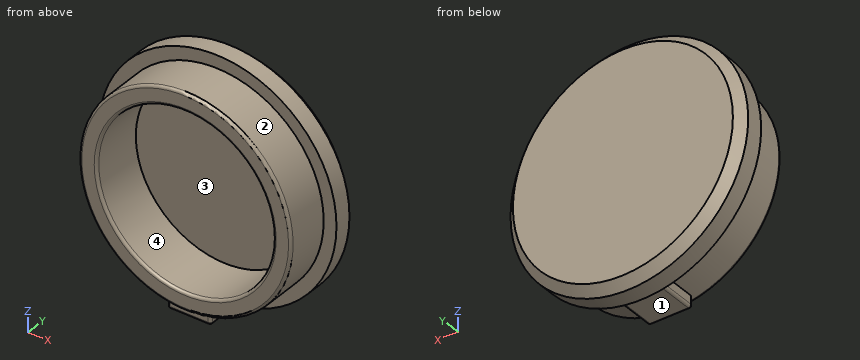
```python
from build123d import *

# Parameters (mm, degrees)
F0_R          = 12
F0_R_2        = 10
F1_DEPTH      = 6
F2_R          = 13.45
F3_DEPTH      = 1
F3_DEPTH_BACK = 2
F4_R          = 10
F5_DEPTH      = 6
F6_W          = 4.9
F6_H          = 2
F7_DEPTH      = 5.4
F8_SIZE       = 1
F9_R          = 0.3
F10_R         = 0.3


with BuildPart() as f1:
    # F0 (on Front) → F1 (new body)
    with BuildSketch(Plane.XZ):
        Circle(F0_R)
        Circle(F0_R_2, mode=Mode.SUBTRACT)
    extrude(amount=F1_DEPTH)

    # F2 (on Front) → F3 (join, two sides)
    with BuildSketch(Plane.XZ) as f3_sk:
        Circle(F2_R)
    extrude(amount=F3_DEPTH)
    extrude(f3_sk.sketch, amount=-F3_DEPTH_BACK)

    # F4 (on Front) → F5 (cut, through all)
    with BuildSketch(Plane.XZ):
        Circle(F4_R)
    extrude(amount=F5_DEPTH, mode=Mode.SUBTRACT)

    # F6 (on Front) → F7 (join)
    with BuildSketch(Plane.XZ):
        with Locations((0, -12)):
            Rectangle(F6_W, F6_H)
    extrude(amount=F7_DEPTH)

    # F8
    f8_edges = [f1.edges().sort_by_distance(p)[0] for p in [
        (-13.45, 2, 0),
    ]]
    chamfer(f8_edges, length=F8_SIZE)

    # F9
    f9_edges = [f1.edges().sort_by_distance(p)[0] for p in [
        (-2.45, -3.2, -13),
        (0, -5.4, -13),
        (2.45, -3.2, -13),
        (-2.45, -5.4, -12.373617),
        (2.45, -5.4, -12.373617),
    ]]
    fillet(f9_edges, radius=F9_R)

    # F10
    f10_edges = [f1.edges().sort_by_distance(p)[0] for p in [
        (-12, -6, 0),
        (-10, -6, 0),
    ]]
    fillet(f10_edges, radius=F10_R)


solid = f1.part
```
Geometry check sheet. Reference: the model listing, model coordinates, mm. Face numbers are marked on the shaded views. Round coordinates to 2 decimals unless told otherwise and drop trailing zeros. Order: outer loops, then holes, each group sorted by start corner. A loop starts at its lowest first (then second) coordinate and runs counter-clockwise, first axis right, second up. Notation, with made-up numbers: (-7, 68.5) - (23, 68.5) arc R19 cw to (23, 101.5) - close; hole circle Ø3 at (47.5, 34). An arc over 180 degrees is marked (long way). Use a Markdown table: item, result. Add a question column.
1) Mould release check, pull along X, two halves, no side actions. Record for the marked faces 1, 2, 3 and 4: released by +X, released by -X, zero draft, split by the parting line, or undercut.
2) Thickness scan on line 1 along Z through (x, y) = (0, -4.1); line 2 along Y through (x, z) = (11.5, -4.5); line 3 along X through (y, z) = (-1.25, -12.5). Record the ranges inside material, lowest first.
3) Section check B-B (y = -4.5). Record the cut outline in (x, z).
4) Section check C-C (z = 0). Record the cut outline in (x, y), then the cut area to 3 significant figures.
5) Gauge pin test, flat ends, axial feed: P1, Ø2, axis at y = -2.5, z = 8, coming from the -X side; P2, Ø3.5, axis at x = -0.5, y = -3.5, coming from the -Z side; P3, Ø0.8, axis at y = -2.5, z = -12.5, coming from the -X side. Record the tip position at first contact, or that the pin passes through.
6) Section check A-A (x = 0). Record the cut outline in (y, z), then the cut area to 3 significant figures.
Established:
| question | item | result |
|---|---|---|
| 1 | face 1 | zero draft |
| 1 | face 2 | split by the parting line |
| 1 | face 3 | undercut |
| 1 | face 4 | undercut |
| 2 | line 1 | -13 to -10, 10 to 12 |
| 2 | line 2 | -1 to 2 |
| 2 | line 3 | -2.45 to 2.45 |
| 3 | outline | (-2.45, -12.7) arc R0.3 ccw to (-2.15, -13) - (2.15, -13) arc R0.3 ccw to (2.45, -12.7) - (2.45, -11.75) arc R12 ccw (long way) to (-2.45, -11.75) - close; hole circle Ø20 at (0, 0) |
| 4 | outline | (-13.45, -1) - (-12, -1) - (-12, -5.7) arc R0.3 ccw to (-11.7, -6) - (-10.3, -6) arc R0.3 ccw to (-10, -5.7) - (-10, 0) - (10, 0) - (10, -5.7) arc R0.3 ccw to (10.3, -6) - (11.7, -6) arc R0.3 ccw to (12, -5.7) - (12, -1) - (13.45, -1) - (13.45, 1) - (12.45, 2) - (-12.45, 2) - (-13.45, 1) - close |
| 4 | area | 79.6 mm2 |
| 5 | P1 | x = -9.75 |
| 5 | P2 | z = -13 |
| 5 | P3 | x = -2.45 |
| 6 | outline | (-6, -11.7) arc R0.3 ccw to (-5.7, -12) - (-5.4, -12) - (-5.4, -12.7) arc R0.3 ccw to (-5.1, -13) - (-1, -13) - (-1, -13.45) - (1, -13.45) - (2, -12.45) - (2, 12.45) - (1, 13.45) - (-1, 13.45) - (-1, 12) - (-5.7, 12) arc R0.3 ccw to (-6, 11.7) - (-6, 10.3) arc R0.3 ccw to (-5.7, 10) - (0, 10) - (0, -10) - (-5.7, -10) arc R0.3 ccw to (-6, -10.3) - close |
| 6 | area | 84.0 mm2 |
